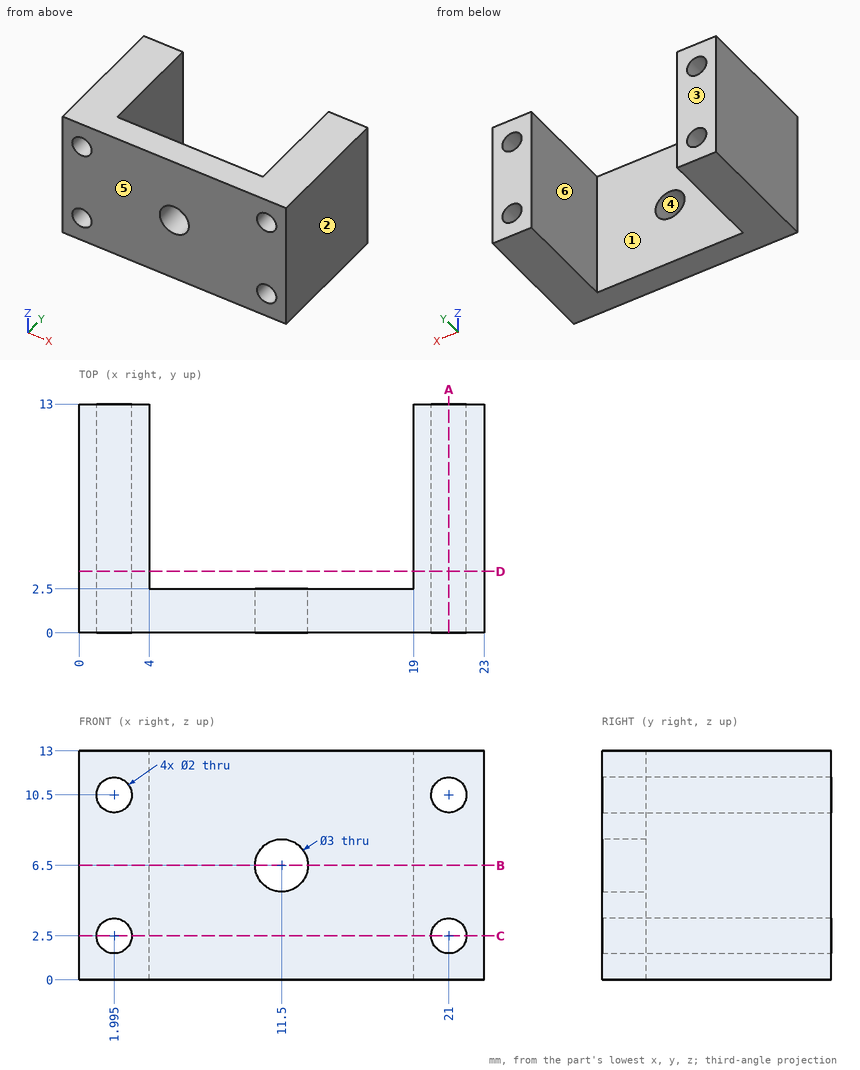
Job drawing, mm, ordinate dimensions from the low corner. One solid piece. A direction names the side the tool comes from. Coordinates: 2 decimals unless noted, no trailing zeros. Loops run counter-clockwise (first coordinate to the right, second up) from the corner with the lowest first, then second, coordinate; pieces in that order, holes last. Notation, with made-up numbers: (56.25, 75) - (80.25, 75) arc R20 ccw to (80.25, 99) - close; hole circle Ø5 at (44.25, 28). An arc over 180 degrees is marked (long way). Answer as a JSON object with one key per item and string values. Group by question number.
(1) Cut at A-A (x = 21). Give the cut face in (y, z).
(2) Cut at D-D (y = 3.5). Give the cut face in (x, z) (3 decimals).
(3) Probe line 1 along X through (y, z) = (10, 10.5) (3 decimals); line 2 along X through (y, z) = (11.5, 5); line 3 along Z through (x, y) = (1.25, 5). List the from-to ranges inside material, lowest first.
(4) Cut at C-C (z = 2.5). Give the cut face in (x, y) (3 decimals), then the cut area to 3 significant figures.
(5) Flat gauge pin, fed straight in: pin 1 (3.5 mm diameter, centred on x = 11.5, z = 6.5, fed in from +Y). Where does the tip first touch, or does it go through?
(6) Cut at B-B (z = 6.5). Give the cut face in (x, y), then the cut area to 3 significant figures.
(7) Two-plate mould, pull along X, no slides. Class the marked faces 1, 2, 3 and 4: released by +X, released by -X, zero draft, split by the parting line, or undercut.
(8) Tool access for the marked faces 5 and 6: list every direction of +Z, -Z, +X, -X, +Y, -Y with a clear straight run to the whole face (end or side of a thin tool).
Geometry says:
{
 "1": {"outline": "(0, 0) - (13, 0) - (13, 1.5) - (0, 1.5) - close; (0, 3.5) - (13, 3.5) - (13, 9.5) - (0, 9.5) - close; (0, 11.5) - (13, 11.5) - (13, 13) - (0, 13) - close"},
 "2": {"outline": "(0, 0) - (4, 0) - (4, 13) - (0, 13) - close; (19, 0) - (23, 0) - (23, 13) - (19, 13) - close; hole circle Ø2 at (1.995, 2.5); hole circle Ø2 at (1.995, 10.5); hole circle Ø2 at (21, 2.5); hole circle Ø2 at (21, 10.5)"},
 "3": {"line 1": "x = 0 to 0.995, 2.995 to 4, 19 to 20, 22 to 23", "line 2": "x = 0 to 4, 19 to 23", "line 3": "z = 0 to 1.83, 3.17 to 9.83, 11.17 to 13"},
 "4": {"outline": "(0, 0) - (0.995, 0) - (0.995, 13) - (0, 13) - close; (2.995, 0) - (20, 0) - (20, 13) - (19, 13) - (19, 2.5) - (4, 2.5) - (4, 13) - (2.995, 13) - close; (22, 0) - (23, 0) - (23, 13) - (22, 13) - close", "area": "89.5 mm^2"},
 "5": {"pin 1": "stops at y = 2.5"},
 "6": {"outline": "(0, 0) - (10, 0) - (10, 2.5) - (4, 2.5) - (4, 13) - (0, 13) - close; (13, 0) - (23, 0) - (23, 13) - (19, 13) - (19, 2.5) - (13, 2.5) - close", "area": "134 mm^2"},
 "7": {"face 1": "undercut", "face 2": "released by +X", "face 3": "zero draft", "face 4": "undercut"},
 "8": {"face 5": "+Z, -Z, +X, -X, -Y", "face 6": "+Z, -Z, +Y"}
}
